Here's the drawing with two shaded views (mm, measured from the low corner). I have some questions. Give positions to 0.01 mm unless a question says otherwise; leave off trailing zeros. Write each loop counter-clockwise with the first axis right and the second up, starting at its lowest first coordinate (ties: lowest second). Pieces come first, ordered by that corner, then holes. Notation, with made-up numbers: (-9.75, -20.75) -> (-3.75, -20.75) arc R24 cw to (-3.75, -7.75) -> close; hole circle Ø11 at (75, 78.5). An arc over 180 degrees is marked (long way). One line per item, written item: value.
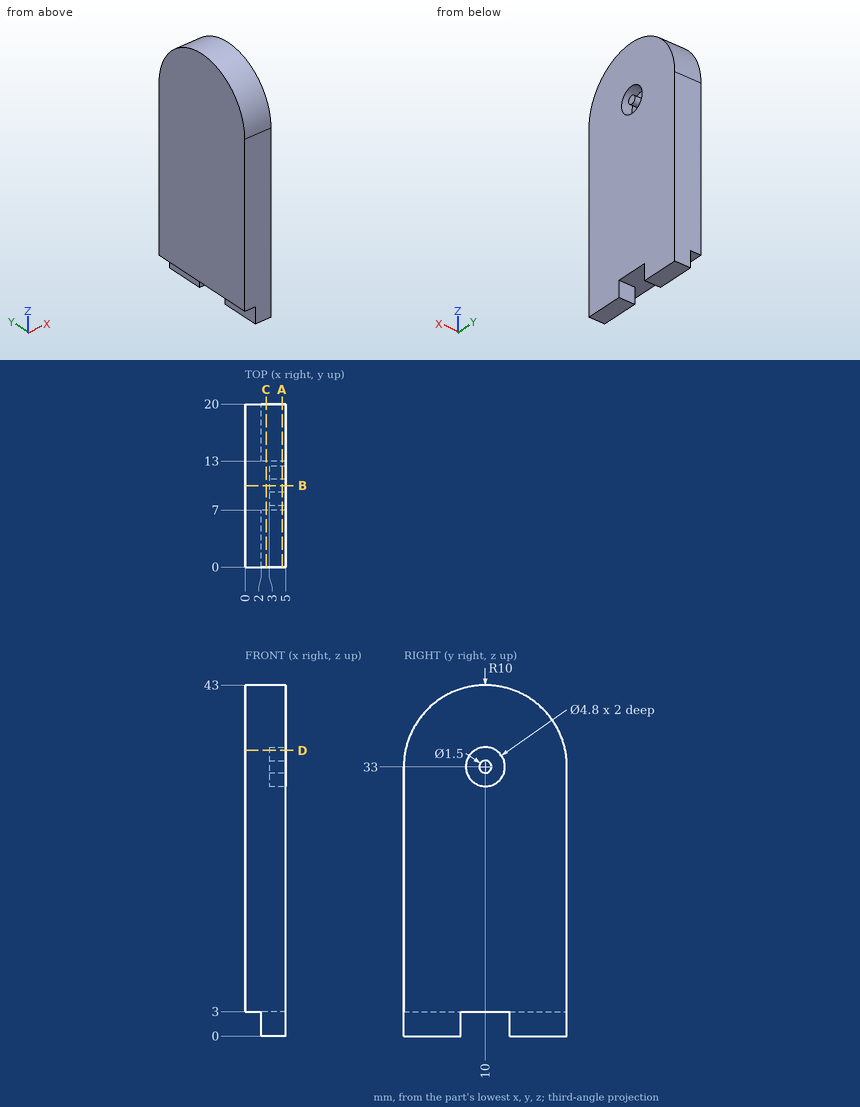
1) If we section it at D-D (z = 35): Write out the boundary of the cut face in (x, y).
Answer list:
outline: (0, 0.2) -> (5, 0.2) -> (5, 8.67) -> (3, 8.67) -> (3, 11.33) -> (5, 11.33) -> (5, 19.8) -> (0, 19.8) -> close
2) If we section it at C-C (x = 2.6): Write out the boundary of the cut face in (y, z).
Answer list:
outline: (0, 0) -> (7, 0) -> (7, 3) -> (13, 3) -> (13, 0) -> (20, 0) -> (20, 33) arc R10 ccw to (0, 33) -> close
3) If we section it at B-B (y = 10): Write out the boundary of the cut face in (x, z).
Answer list:
outline: (0, 3) -> (5, 3) -> (5, 30.6) -> (3, 30.6) -> (3, 32.25) -> (5, 32.25) -> (5, 33.75) -> (3, 33.75) -> (3, 35.4) -> (5, 35.4) -> (5, 43) -> (0, 43) -> close
4) If we section it at A-A (x = 4.55): Write out the boundary of the cut face in (y, z), and give its area (3 significant figures).
Answer list:
outline: (0, 0) -> (7, 0) -> (7, 3) -> (13, 3) -> (13, 0) -> (20, 0) -> (20, 33) arc R10 ccw to (0, 33) -> close; circle Ø1.5 at (10, 33); hole circle Ø4.8 at (10, 33)
area: 783 mm^2
5) I need wall thicknesses on L1, parallel to Z at x = 3.75, y = 10; L2, parallel to Z at x = 1.4, y = 5.5; L3, parallel to Z at x = 4.3, y = 14. Which ranges of each line are inside material? Lowest first, please.
Answer list:
L1: z = 3 to 30.6, 32.25 to 33.75, 35.4 to 43
L2: z = 3 to 41.93
L3: z = 0 to 42.17
6) Will these pins go through, and if not, where does the flat tip stop? pin 1 (1 mm diameter, centred on x = 2, y = 9.5, fed in from +Z); pin 2 (2.5 mm diameter, centred on y = 18, z = 1, fed in from -X).
Answer list:
pin 1: stops at z = 43
pin 2: stops at x = 2
